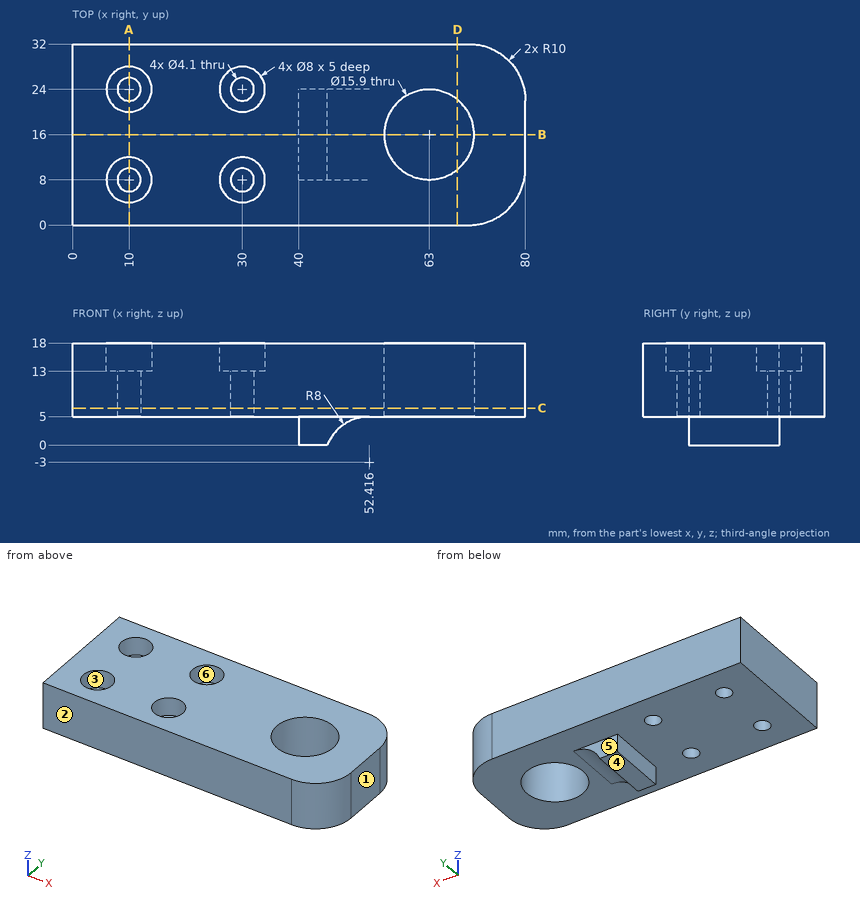
Print and shaded views of the part. All mm, measured from the part's lowest x, y and z. A direction names the side the tool comes from. Give positions to 0.01 mm unless a question says otherwise; leave off trailing zeros. Order: outer loops, then holes, each group sorted by start corner. A loop starts at its lowest first (then second) coordinate and runs counter-clockwise, first axis right, second up. Notation, with made-up numbers: (-24.75, 51) - (-2.75, 51) arc R30 cw to (-2.75, 80) - close; hole circle Ø10 at (-2.5, -20). An arc over 180 degrees is marked (long way). Use a Markdown table: item, result.
1) Flat gauge pins, fed straight in: P1, Ø2.5, axis at x = 10, y = 22.5, coming from the +Z side; P2, Ø3.5, axis at x = 10, y = 8, coming from the -Z side; P3, Ø3, axis at x = 49, y = 22, coming from the -Z side; P4, Ø9.5, axis at x = 57.5, y = 15.5, coming from the -Z side. Where does each tip first touch, or does it go through?
Checked values:
| item | result |
|---|---|
| P1 | z = 13 |
| P2 | through |
| P3 | z = 3.31 |
| P4 | z = 5 |
2) Probe L1, parallel to Y at x = 10, z = 14.5; L2, parallel to Y at x = 30, z = 10.25; L3, parallel to Z at x = 15.5, y = 23. List the from-to ranges inside material, lowest first. Write a range as from..to.
Checked values:
| item | result |
|---|---|
| L1 | 0..4, 12..20, 28..32 |
| L2 | 0..5.95, 10.05..21.95, 26.05..32 |
| L3 | 5..18 |
3) 3-axis set-ups, long thin cutter, end or side, ignore diameter. For the marked faces 4, 5 and 6: which of +Z, -Z, +X, -X, +Y, -Y reach the whole face in a straight line?
Checked values:
| item | result |
|---|---|
| face 4 | -Z, +X, -X, +Y, -Y |
| face 5 | -Z, +X, -X, +Y |
| face 6 | +Z |
4) Saw through at C-C on z = 6.5. List the corners of the cut face in (x, y).
Checked values:
| item | result |
|---|---|
| outline | (0, 0) - (70, 0) arc R10 ccw to (80, 10) - (80, 22) arc R10 ccw to (70, 32) - (0, 32) - close; hole circle Ø4.1 at (10, 8); hole circle Ø4.1 at (10, 24); hole circle Ø4.1 at (30, 8); hole circle Ø4.1 at (30, 24); hole circle Ø15.9 at (63, 16) |
5) Saw through at B-B on y = 16. List the corners of the cut face in (x, z).
Checked values:
| item | result |
|---|---|
| outline | (0, 5) - (40, 5) - (40, 0) - (45, 0) arc R8 cw to (52.42, 5) - (55.05, 5) - (55.05, 18) - (0, 18) - close; (70.95, 5) - (80, 5) - (80, 18) - (70.95, 18) - close |
6) Saw through at D-D on x = 68. List the corners of the cut face in (y, z), plus the area to 3 significant figures.
Checked values:
| item | result |
|---|---|
| outline | (0, 5) - (9.82, 5) - (9.82, 18) - (0, 18) - close; (22.18, 5) - (32, 5) - (32, 18) - (22.18, 18) - close |
| area | 255 mm² |
7) Saw through at A-A on x = 10. List the corners of the cut face in (y, z).
Checked values:
| item | result |
|---|---|
| outline | (0, 5) - (5.95, 5) - (5.95, 13) - (4, 13) - (4, 18) - (0, 18) - close; (10.05, 5) - (21.95, 5) - (21.95, 13) - (20, 13) - (20, 18) - (12, 18) - (12, 13) - (10.05, 13) - close; (26.05, 5) - (32, 5) - (32, 18) - (28, 18) - (28, 13) - (26.05, 13) - close |
8) Two-plate mould, pull along X, no slides. Class the marked faces 1, 2 and 3: +X half, -X half, draft (parallel to the pull), parting line (faces both ways), or undercut.
Checked values:
| item | result |
|---|---|
| face 1 | +X half |
| face 2 | draft |
| face 3 | undercut |
